```python
from build123d import *

# Parameters (mm, degrees)
SKETCH1_R           = 9
BOSS_EXTRUDE1_DEPTH = 2.5
BOSS_EXTRUDE2_START = 131
BOSS_EXTRUDE2_DEPTH = 131


with BuildPart() as part:
    # Sketch1 → Boss-Extrude1 (new, symmetric)
    with BuildSketch(Plane.XY):
        with BuildLine():
            Line((-5, 13.829316686), (-5, 66))
            ThreePointArc((-5, 66), (-3.828427125, 68.828427125), (-1, 70))
            Line((-1, 70), (1, 70))
            ThreePointArc((1, 70), (3.828427125, 68.828427125), (5, 66))
            Line((5, 66), (5, 13.829316686))
            ThreePointArc((5, 13.829316686), (5.483803708, 11.922391507), (6.818181818, 10.476755065))
            ThreePointArc((6.818181818, 10.476755065), (0, -12.5), (-6.818181818, 10.476755065))
            ThreePointArc((-6.818181818, 10.476755065), (-5.483803708, 11.922391507), (-5, 13.829316686))
        make_face()
        Circle(SKETCH1_R, mode=Mode.SUBTRACT)
    boss_extrude1 = extrude(amount=BOSS_EXTRUDE1_DEPTH, both=True)

    # Sketch2 → Boss-Extrude2 (add)
    with BuildSketch(Plane.XY.offset(2.5).offset(BOSS_EXTRUDE2_START)):
        with BuildLine():
            Line((-5, 66), (-5, 61.401358418))
            Line((-5, 61.401358418), (5, 61.401358418))
            Line((5, 61.401358418), (5, 66))
            ThreePointArc((5, 66), (3.828427125, 68.828427125), (1, 70))
            Line((1, 70), (-1, 70))
            ThreePointArc((-1, 70), (-3.828427125, 68.828427125), (-5, 66))
        make_face()
    extrude(amount=-BOSS_EXTRUDE2_DEPTH)

    # Mirror1: Boss-Extrude1 across plane
    add(boss_extrude1.mirror(Plane.XY.offset(68)))


solid = part.part
```
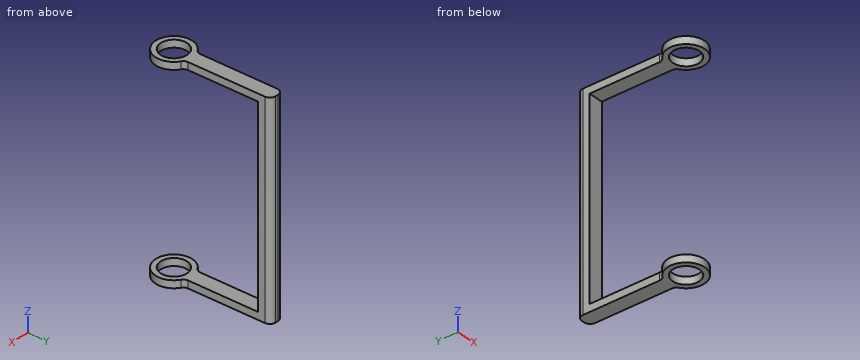
Design review of the part built by this model. Coordinates are the model's own, in mm. Coordinates: 2 decimals unless noted, no trailing zeros. Order: outer loops, then holes, each group sorted by start corner. A loop starts at its lowest first (then second) coordinate and runs counter-clockwise, first axis right, second up. Notation, with made-up numbers: (85, 21.5) -> (122, 21.5) arc R20 cw to (122, 25.5) -> close; hole circle Ø9 at (11, 60). An arc over 180 degrees is marked (long way). One line per item, written item: value. Start each with the question number.
Q1. Insertion check: pin 1 Ø2 at (x, z) = (2.5, 124) entering from +Y; pin 2 Ø8 at (x, z) = (0.5, 96.5) entering from -Y. Each pin has a flat end and moves straight along its axis. Give the tip position at first contact, or say it passes through.
Q2. Take a section at B-B, the plane x = 2.5. State the section outline as (y, z) points.
Q3. Take a section at C-C, the plane y = 0. State the section outline as (x, z) points.
Q4. Take a section at A-A, the plane y = 15.5. State the section outline as (x, z) points.
Q5. For probe 1 along Y at (x, z) = (0, 135.4); probe 2 along Z at (x, y) = (0.75, 21.5); probe 3 along Y at (x, z) = (1.5, 68), list the stretches that pass through material, from the lowest coordinate up.
Q6. Take a section at D-D, the plane z = 83.5. State the section outline as (x, y) points, then the cut area to 3 significant figures.
Values follow:
1. pin 1: stops at y = 69.97
1. pin 2: stops at y = 61.4
2. outline: (-12.25, -2.5) -> (-8.65, -2.5) -> (-8.65, 2.5) -> (-12.25, 2.5) -> close; (-12.25, 133.5) -> (-8.65, 133.5) -> (-8.65, 138.5) -> (-12.25, 138.5) -> close; (8.65, -2.5) -> (69.71, -2.5) -> (69.71, 138.5) -> (8.65, 138.5) -> (8.65, 133.5) -> (61.4, 133.5) -> (61.4, 2.5) -> (8.65, 2.5) -> close
3. outline: (-12.5, -2.5) -> (-9, -2.5) -> (-9, 2.5) -> (-12.5, 2.5) -> close; (-12.5, 133.5) -> (-9, 133.5) -> (-9, 138.5) -> (-12.5, 138.5) -> close; (9, -2.5) -> (12.5, -2.5) -> (12.5, 2.5) -> (9, 2.5) -> close; (9, 133.5) -> (12.5, 133.5) -> (12.5, 138.5) -> (9, 138.5) -> close
4. outline: (-5, -2.5) -> (5, -2.5) -> (5, 2.5) -> (-5, 2.5) -> close; (-5, 133.5) -> (5, 133.5) -> (5, 138.5) -> (-5, 138.5) -> close
5. probe 1: y = -12.5 to -9, 9 to 70
5. probe 2: z = -2.5 to 2.5, 133.5 to 138.5
5. probe 3: y = 61.4 to 69.97
6. outline: (-5, 61.4) -> (5, 61.4) -> (5, 66) arc R4 ccw to (1, 70) -> (-1, 70) arc R4 ccw to (-5, 66) -> close
6. area: 79.1 mm2
